Design review of the part built by this model. Coordinates are the model's own, in mm. Face numbers are marked on the shaded views. A direction names the side the tool comes from. Give positions to 0.01 mm unless a question says otherwise; leave off trailing zeros. Loops run counter-clockwise (first coordinate to the right, second up) from the corner with the lowest first, then second, coordinate; pieces in that order, holes last. Notation, with made-up numbers: (-7, 68.25) -> (24, 68.25) arc R21 ccw to (24, 93.25) -> close; hole circle Ø3 at (78.5, 60). An arc over 180 degrees is marked (long way). Answer as CSV lines item,"result".
Autodesk Inventor part; units mm, degrees
ref_plane "YZ Plane" through (0, 0, 0) normal (1, 0, 0) x (0, 1, 0)
ref_plane "XZ Plane" through (0, 0, 0) normal (0, 1, 0) x (-1, 0, 0)
ref_plane "XY Plane" through (0, 0, 0) normal (0, 0, 1) x (1, 0, 0)
sketch "Skizze1" plane through (0, 0, 0) normal (1, 0, 0) x (0, 1, 0)
  line L0 (12.5, 3) -> (12.5, -3) construction
  line L1 (-12.5, -3) -> (-12.5, 3) construction
  line L2 (6, 26.2642) -> (6, -26.2642) construction
  line L3 (-6, -26.2642) -> (-6, 26.2642) construction
  line L4 (14, 26.2642) -> (14, -26.2642) construction
  line L5 (-14, -26.2642) -> (-14, 26.2642) construction
  line L6 (23.5, 26.2642) -> (23.5, -26.2642) construction
  line L7 (-23.5, -26.2642) -> (-23.5, 26.2642) construction
  line L8 (12.5, -3) -> (0, -3)
  line L9 (0, -3) -> (0, -8)
  line L10 (0, -8) -> (6, -8)
  line L11 (6, -8) -> (6, -13)
  line L12 (6, -13) -> (14, -13)
  line L13 (14, -13) -> (14, -10)
  line L14 (25, 26.2642) -> (25, -26.2642) construction
  line L15 (-25, -26.2642) -> (-25, 26.2642) construction
  line L16 (14, -10) -> (23.5, -10)
  line L17 (23.5, -10) -> (23.5, -7)
  line L18 (23.5, -7) -> (25, -7)
  line L19 (25, -7) -> (25, 0)
  line L20 (12.5, -3) -> (12.5, 0)
  line L21 (25, 0) -> (12.5, 0)
  point P0 (0, 0)
  dimension "d1" = 6
  dimension "d5" = 5
  dimension "d6" = 6
  dimension "d7" = 5
  dimension "d8" = 3
  dimension "d9" = 47
  dimension "d10" = 50
  dimension "d11" = 3
revolve "Umdrehung1" add sketch "Skizze1" angle 360 about axis through (0, 0, -3) along (0, 0, -1)
sketch "Skizze2" plane through (0, 0, -10) normal (0, 0, -1) x (-1, 0, 0)
  circle A0 centre (0, 0) radius 18 construction
  circle A1 centre (0, 18) radius 2
  dimension "d13" = 36
  dimension "d14" = 4
extrude "Extrusion1" cut sketch "Skizze2" against normal up to surface (10 mm away)
pattern_circular "Runde Anordnung1" count 4 over 360 about axis through (0, 0, -10.5) along (0, 0, -1) of "Extrusion1"
sketch "Skizze3" plane through (0, 0, -13) normal (0, 0, -1) x (-1, 0, 0)
  line L0 (0, 0) -> (-21.5822, 21.5822) construction
  line L1 (0, 0) -> (30.5219, 0) construction
  line L2 (-16.2635, 9.1924) -> (-9.1924, 16.2635)
  line L3 (-9.1924, 16.2635) -> (-3.5355, 10.6066)
  line L4 (-3.5355, 10.6066) -> (-10.6066, 3.5355)
  line L5 (-10.6066, 3.5355) -> (-16.2635, 9.1924)
  circle A0 centre (0, 0) radius 14
  line L6 (-16.2635, 9.1924) -> (-3.5355, 10.6066) construction
  line L7 (-9.1924, 16.2635) -> (-10.6066, 3.5355) construction
  point P0 (-9.8995, 9.8995)
  point P1 (-5.7111, 12.7822)
  point P2 (-12.7822, 5.7111)
  dimension "d20" = 135
  dimension "d21" = 10
  dimension "d22" = 8
extrude "Extrusion2" cut sketch "Skizze3" against normal up to surface (3 mm away) contours A0 L3 L4 L5 picked at (-7.5887, 8.3902)
fillet "Rundung1" radius 1.5 2 edges at (3.5355, 10.6066, -11.5) (10.6066, 3.5355, -11.5)
fillet "Rundung2" radius 0.5 3 edges at (0, -12.5, 0) (0, -12.5, -3) (0, -25, 0)
properties part number "sf_Cylinder_Front_Lid_1"
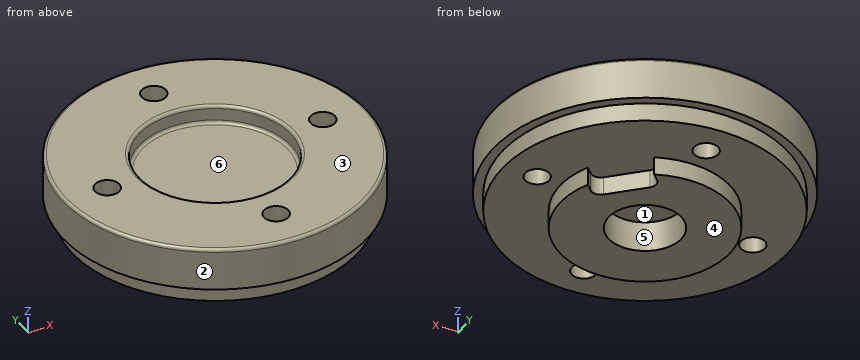
Q1. We need section A-A, the plane y = 0. State how many separate pieces and enclosed holes the cut face has, and give its area (3 significant figures).
Filled sheet:
separate pieces,"3"
enclosed holes,"0"
area,"360 mm^2"
Q2. For the marked faces 4, 5 and 6, list the 3-axis set-ups (+Z, -Z, +X, -X, +Y, -Y) from which the entire face can be reached by the end or side of a thin tool; tool diameter is ignored.
Filled sheet:
face 4,"-Z, +X, -X, +Y, -Y"
face 5,"-Z"
face 6,"+Z"
Q3. To check wall thickness, follow probe 1 along X at (y, z) = (0, -2.25); probe 2 along X at (y, z) = (0, -10.85); probe 3 along Z at (x, y) = (11, 3). State the ranges of each line that lie inside material, in increasing order. Write a range as from..to.
Filled sheet:
probe 1,"x = -25..-20, -16..-12.5, 12.5..16, 20..25"
probe 2,"x = -14..-6, 6..14"
probe 3,"z = -13..-3"
Q4. We need section D-D, the plane z = -1.75. State the section outline as (x, y) points.
Filled sheet:
outline,"circle Ø50 at (0, 0); hole circle Ø4 at (-18, 0); hole circle Ø25 at (0, 0); hole circle Ø4 at (0, -18); hole circle Ø4 at (0, 18); hole circle Ø4 at (18, 0)"
Q5. The part is to be moulded in two halves that separate along X. For the marked faces 1, 2 and 3, say which applies: pulls with the +X half, pulls with the -X half, needs draft (parallel to the pull), parting line crosses it, or undercut.
Filled sheet:
face 1,"undercut"
face 2,"parting line crosses it"
face 3,"needs draft"
Q6. Clearance check with flat-ended pins moving along their axes: pin 1 Ø4.5 at (x, y) = (18, 0) entering from +Z; pin 2 Ø6 at (x, y) = (-2, 1.5) entering from -Z; pin 3 Ø3.5 at (x, y) = (0, 18) entering from -Z; pin 4 Ø5 at (x, z) = (6, -5) entering from -Y. State where each tip first meets the part, or that it passes through.
Filled sheet:
pin 1,"stops at z = 0"
pin 2,"stops at z = -8"
pin 3,"passes through"
pin 4,"stops at y = -24.75"
Q7. We need section C-C, the plane z = -11.75. State the section outline as (x, y) points, and give its area (3 significant figures).
Filled sheet:
outline,"(4.6, 9.55) arc R1.5 cw to (4.6, 11.67) -> (5.71, 12.78) arc R14 ccw (long way) to (12.78, 5.71) -> (11.67, 4.6) arc R1.5 cw to (9.55, 4.6) -> close; hole circle Ø12 at (0, 0)"
area,"467 mm^2"
